For this review, use the dimensioned drawing (mm, ordinates from the lowest corner) and the shaded views. A direction names the side the tool comes from. Round coordinates to 2 decimals unless told otherwise and drop trailing zeros. Write each loop counter-clockwise with the first axis right and the second up, starting at its lowest first coordinate (ties: lowest second). Pieces come first, ordered by that corner, then holes.
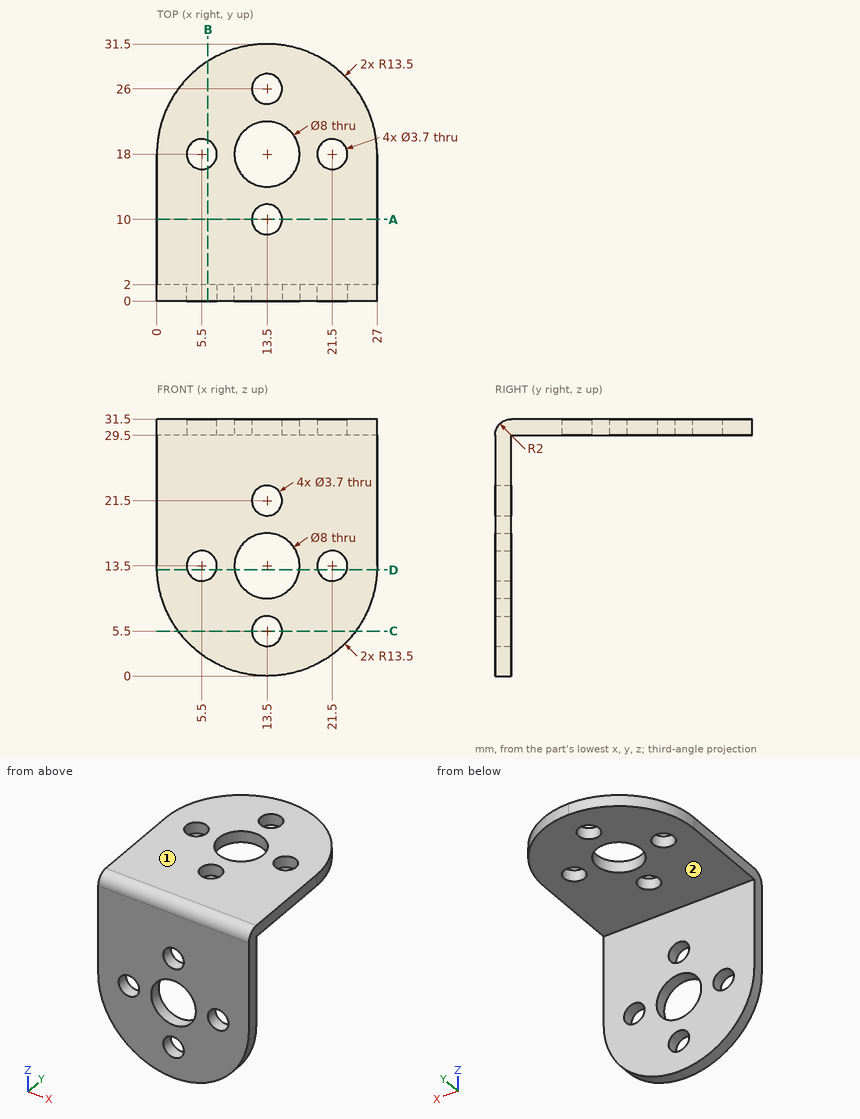
(1) We need section D-D, the plane z = 13. Give the boundary of the cut face in (x, y), and give its area (3 significant figures).
Geometry check:
outline: (0.01, 0) - (3.72, 0) - (3.72, 2) - (0.01, 2) - close; (7.28, 0) - (9.53, 0) - (9.53, 2) - (7.28, 2) - close; (17.47, 0) - (19.72, 0) - (19.72, 2) - (17.47, 2) - close; (23.28, 0) - (26.99, 0) - (26.99, 2) - (23.28, 2) - close
area: 23.8 mm2
(2) We need section A-A, the plane y = 10. Give the boundary of the cut face in (x, z), and give its area (3 significant figures).
Geometry check:
outline: (0, 29.5) - (11.65, 29.5) - (11.65, 31.5) - (0, 31.5) - close; (15.35, 29.5) - (27, 29.5) - (27, 31.5) - (15.35, 31.5) - close
area: 46.6 mm2
(3) For the marked faces 1 and 2, list the 3-axis set-ups (+Z, -Z, +X, -X, +Y, -Y) from which the entire face can be reached by the end or side of a thin tool; tool diameter is ignored.
Geometry check:
face 1: +Z, +X, -X, +Y, -Y
face 2: -Z, +X, -X, +Y
(4) For pin 1 Ø6.5 at (x, z) = (13.5, 13.5) entering from +Y; pin 2 Ø4 at (x, z) = (23, 25) entering from +Y; pin 3 Ø6 at (x, y) = (21.5, 18) entering from +Z; pin 4 Ø2 at (x, y) = (3.5, 28) entering from -Z, all flat-tipped, find the tip position at first contact; note any pin that passes through.
Geometry check:
pin 1: passes through
pin 2: stops at y = 2
pin 3: stops at z = 31.5
pin 4: stops at z = 29.5
(5) For line 1 along Z through (x, y) = (10.5, 15); line 2 along Y through (x, z) = (17.5, 29); line 3 along X through (y, z) = (1, 5), list the stretches that pass through material, from the lowest coordinate up.
Geometry check:
line 1: z = 29.5 to 31.5
line 2: y = 0 to 2
line 3: x = 3.01 to 11.72, 15.28 to 23.99
(6) We need section B-B, the plane x = 6.25. Give the boundary of the cut face in (y, z).
Geometry check:
outline: (0, 2.11) - (2, 2.11) - (2, 11.81) - (0, 11.81) - close; (0, 15.19) - (2, 15.19) - (2, 29.5) - (16.31, 29.5) - (16.31, 31.5) - (2, 31.5) arc R2 ccw to (0, 29.5) - close; (19.69, 29.5) - (29.39, 29.5) - (29.39, 31.5) - (19.69, 31.5) - close
(7) We need section C-C, the plane z = 5.5. Give the boundary of the cut face in (x, y), and give its area (3 significant figures).
Geometry check:
outline: (2.63, 0) - (11.65, 0) - (11.65, 2) - (2.63, 2) - close; (15.35, 0) - (24.37, 0) - (24.37, 2) - (15.35, 2) - close
area: 36.1 mm2
